```python
from build123d import *

# Parameters (mm, degrees)
BOSS_EXTRU_1_DEPTH      = 60
ESQUISSE2_R             = 2
ENL_V_MAT_EXTRU_1_DEPTH = 10
ESQUISSE3_R             = 1.75
BOSS_EXTRU_2_DEPTH      = 9


with BuildPart() as part:
    # Esquisse1 → Boss.-Extru.1 (new body)
    with BuildSketch(Plane(origin=(0, 0, 0), x_dir=(1, 0, 0), z_dir=(0, 1, 0))):
        Polygon((3.655828371, -1.722861646), (3.319956139, 2.304609418), (-0.335872233, 4.027471065), (-3.655828371, 1.722861646), (-3.319956139, -2.304609418), (0.335872233, -4.027471065), align=None)
    extrude(amount=BOSS_EXTRU_1_DEPTH)

    # Esquisse2 → Enlèv. mat.-Extru.1 (cut)
    with BuildSketch(Plane.XZ):
        with Locations(Location((0, 0, 0), (0, 0, 270))):
            Circle(ESQUISSE2_R)
    extrude(amount=-ENL_V_MAT_EXTRU_1_DEPTH, mode=Mode.SUBTRACT)

    # Esquisse3 → Boss.-Extru.2 (add)
    with BuildSketch(Plane(origin=(0, 60, 0), x_dir=(1, 0, 0), z_dir=(0, 1, 0))):
        with Locations(Location((0, 0, 0), (0, 0, 270))):
            Circle(ESQUISSE3_R)
    extrude(amount=BOSS_EXTRU_2_DEPTH)


solid = part.part
```
Could you check a few things on this model? Use its own coordinates, in mm. A direction names the side the tool comes from. Round coordinates to 2 decimals unless told otherwise and drop trailing zeros. Loops run counter-clockwise (first coordinate to the right, second up) from the corner with the lowest first, then second, coordinate; pieces in that order, holes last.
Q1. I want a section at C-C (y = 41.5). Write out the boundary of the cut face in (x, z), and give its area (3 significant figures).
Q2. Thinking about a two-plate mould opening in X: for faces 4 (the flat face through (0, 10, 0)), 5 (the flat face through (-1, 0, -2)), 6 (the flat face through (-3.49, 29.58, 0.26)), which applies, pulls with the +X half, pulls with the -X half, needs draft (parallel to the pull), parting line crosses it, or undercut?
Q3. I want a section at B-B (z = -1). Write out the boundary of the cut face in (x, y), and give its area (3 significant figures).
Q4. On a 3-axis mill with a long thin cutter (end or side, diameter ignored), from which of +Z, -Z, +X, -X, +Y, -Y can I reach the whole of each face in a straight line? I mean faces 1 (the flat face through (1.518, 29.58, -3.154)), 2 (the cylindrical face through (-2, 5, 0)), 3 (the flat face through (0, 60, -2)). Say none if no direction works.
Q5. Please list where these lines run through material, in increasing order: L1, parallel to Y at x = 1.5, z = -0.25; L2, parallel to Y at x = 0.75, z = 2.5; L3, parallel to X at y = 4.25, z = 0.
Q6. I want a section at A-A (y = 7). Write out the boundary of the cut face in (x, z).
Q7. For P1, Ø2, axis at x = 0.5, z = -0.5, coming from the -Y side; P2, Ø4, axis at x = 2.5, y = 31, coming from the +Z side; P3, Ø2, axis at x = -2, y = 16.5, coming from the -Z side, each with a flat end and sliding along its axis, tell me the tip position at first contact or that it passes through.
Answer below:
1. outline: (-3.66, -1.72) - (-0.34, -4.03) - (3.32, -2.3) - (3.66, 1.72) - (0.34, 4.03) - (-3.32, 2.3) - close
1. area: 42.4 mm2
2. face 4: undercut
2. face 5: needs draft
2. face 6: pulls with the -X half
3. outline: (-3.6, 0) - (-1.73, 0) - (-1.73, 10) - (1.73, 10) - (1.73, 0) - (3.43, 0) - (3.43, 60) - (1.44, 60) - (1.44, 69) - (-1.44, 69) - (-1.44, 60) - (-3.6, 60) - close
3. area: 413 mm2
4. face 1: -Z, +X, +Y, -Y
4. face 2: -Y
4. face 3: +Y
5. L1: y = 10 to 69
5. L2: y = 0 to 60
5. L3: x = -3.51 to -2, 2 to 3.51
6. outline: (-3.66, -1.72) - (-0.34, -4.03) - (3.32, -2.3) - (3.66, 1.72) - (0.34, 4.03) - (-3.32, 2.3) - close; hole circle Ø4 at (0, 0)
7. P1: stops at y = 10
7. P2: stops at z = 3.91
7. P3: stops at z = -3.57
